Model file for the job. Use its own axes, mm. Face numbers are marked on the shaded views. A direction names the side the tool comes from. Round coordinates to 2 decimals unless told otherwise and drop trailing zeros. Loops run counter-clockwise (first coordinate to the right, second up) from the corner with the lowest first, then second, coordinate; pieces in that order, holes last. Notation, with made-up numbers: (65.25, -25.75) - (74.25, -25.75) arc R32 cw to (74.25, 9.25) - close; hole circle Ø2 at (18, -6). An arc over 180 degrees is marked (long way). Answer as a JSON object with one key per item and string values.
Autodesk Inventor part; units mm, degrees
ref_plane "YZ Plane" through (0, 0, 0) normal (1, 0, 0) x (0, 1, 0)
ref_plane "XZ Plane" through (0, 0, 0) normal (0, 1, 0) x (-1, 0, 0)
ref_plane "XY Plane" through (0, 0, 0) normal (0, 0, 1) x (1, 0, 0)
sketch "Sketch1" plane through (0, 0, 0) normal (0, 0, 1) x (1, 0, 0)
  line L0 (16, -16) -> (-16, -16)
  line L1 (-16, -16) -> (-16, 16)
  line L2 (-16, 16) -> (16, 16)
  line L3 (16, 16) -> (16, -16)
  line L4 (16, -16) -> (-16, 16) construction
  line L5 (-16, -16) -> (16, 16) construction
  line L6 (14, 14) -> (-14, 14)
  line L7 (-14, 14) -> (-14, -14)
  line L8 (-14, -14) -> (14, -14)
  line L9 (14, -14) -> (14, 14)
  line L10 (20, -20) -> (-20, -20)
  line L11 (-20, -20) -> (-20, 20)
  line L12 (-20, 20) -> (20, 20)
  line L13 (20, 20) -> (20, -20)
  line L14 (-11, 11) -> (11, 11)
  line L15 (11, 11) -> (11, -11)
  line L16 (11, -11) -> (-11, -11)
  line L17 (-11, -11) -> (-11, 11)
  point P0 (0, 0)
  dimension "d0" = 32
  dimension "d1" = 32
  dimension "d2" = 2
  dimension "d10" = 4
  dimension "d12" = 3
extrude "Extrusion1" add sketch "Sketch1" against normal blind 2 contours L9 L8 L7 L6 | L14 L15 L16 L17
extrude "Extrusion2" add sketch "Sketch1" against normal blind 2 from surface at -2 contours L0 L1 L2 L3 | L9 L8 L7 L6 | L14 L15 L16 L17
fillet "Fillet1" radius 4 8 edges at (-16, 16, -3) (16, 16, -3) (-16, -16, -3) (14, -14, -1) (-14, -14, -1) (-14, 14, -1) (14, 14, -1) (16, -16, -3)
pattern_linear "Rectangular Pattern1" count 3 spacing 4 along (0, 0, -1)
extrude "Extrusion3" add sketch "Sketch1" along normal blind 4 contours L0 L1 L2 L3 | L9 L8 L7 L6 | L10 L11 L12 L13 | L14 L15 L16 L17
fillet "Fillet2" radius 5 4 edges at (-20, 20, 2) (20, 20, 2) (-20, -20, 2) (20, -20, 2)
extrude "Extrusion4" cut sketch "Sketch1" against normal through all contours L14 L15 L16 L17
fillet "Fillet3" radius 1 8 edges at (0, 20, 4) (-18.5355, 18.5355, 4) (-20, 0, 4) (-18.5355, -18.5355, 4) (0, -20, 4) (18.5355, -18.5355, 4) (20, 0, 4) (18.5355, 18.5355, 4)
properties part number "PWTR-0123" material "Rubber"
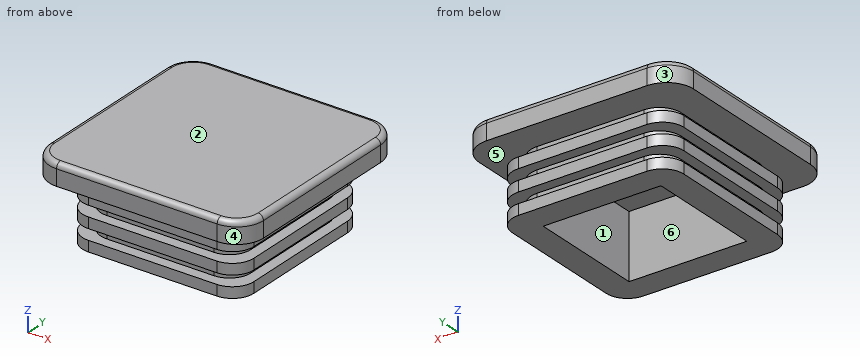
1) Two-plate mould, pull along Y, no slides. Class the marked faces 3, 4, 5 and 6: pulls with the +Y half, pulls with the -Y half, needs draft (parallel to the pull), parting line crosses it, or undercut.
Values follow:
{"face 3": "pulls with the +Y half", "face 4": "pulls with the -Y half", "face 5": "needs draft", "face 6": "undercut"}
2) Slice it at B-B on y = -14.5. List the corners of the cut face in (x, z).
Values follow:
{"outline": "(-20, 0) - (20, 0) - (20, 3) arc R1 ccw to (19, 4) - (-19, 4) arc R1 ccw to (-20, 3) - close; (-15.12, -12) - (15.12, -12) - (15.12, -10) - (-15.12, -10) - close; (-15.12, -8) - (15.12, -8) - (15.12, -6) - (-15.12, -6) - close; (-15.12, -4) - (15.12, -4) - (15.12, -2) - (-15.12, -2) - close"}
3) Probe probe 1 along X at (y, z) = (3, -5); probe 2 along Y at (x, z) = (-5.5, -2.75). List the from-to ranges inside material, lowest first.
Values follow:
{"probe 1": "-14 to -11, 11 to 14", "probe 2": "-16 to -11, 11 to 16"}
4) Drop flat-ended pins along their axis: P1, Ø5, axis at x = -0.5, y = -2, coming from the -Z side; P2, Ø2, axis at x = 5.5, z = -3, coming from the -Y side; P3, Ø0.6, axis at y = -6, z = -10.5, coming from the -X side. Give the stop position or say it passes through.
Values follow:
{"P1": "z = 0", "P2": "y = -16", "P3": "x = -16"}
5) Tool access for the marked faces 1 and 2: list every direction of +Z, -Z, +X, -X, +Y, -Y with a clear straight run to the whole face (end or side of a thin tool).
Values follow:
{"face 1": "-Z", "face 2": "+Z, +X, -X, +Y, -Y"}
6) Slice it at A-A on z = -1.5. List the corners of the cut face in (x, y), then the cut area to 3 significant figures.
Values follow:
{"outline": "(-14, -10) arc R4 ccw to (-10, -14) - (10, -14) arc R4 ccw to (14, -10) - (14, 10) arc R4 ccw to (10, 14) - (-10, 14) arc R4 ccw to (-14, 10) - close; hole (-11, -11) - (11, -11) - (11, 11) - (-11, 11) - close", "area": "286 mm²"}
